```python
from build123d import *

# Parameters (mm, degrees)
F1_DEPTH = 25.4
F2_R     = 3.429
F3_DEPTH = 147.32
F4_W     = 22.8622798618
F4_H     = 12.7
F5_DEPTH = 25.4
F6_DEPTH = 76.2
F8_DEPTH = 25.4
F9_R     = 5.08


with BuildPart() as f1:
    # F0 (on Front) → F1 (new body)
    with BuildSketch(Plane.XZ):
        with BuildLine():
            Line((-25.4, 124.5236706513), (-25.4, 91.1413904513))
            Line((-25.4, 91.1413904513), (-25.4, -91.1413904513))
            Line((-25.4, -91.1413904513), (-25.4, -91.4211095487))
            Line((-25.4, -91.4211095487), (-25.4, -129.4763404513))
            Line((-25.4, -129.4763404513), (-2.5377201382, -129.4763404513))
            Line((-2.5377201382, -129.4763404513), (-2.5377201382, -103.8838730506))
            ThreePointArc((-2.5377201382, -103.8838730506), (-9.8366418496, -99.4730864008), (-12.7, -91.44))
            Line((-12.7, -91.44), (-12.7, 91.44))
            ThreePointArc((-12.7, 91.44), (-9.8366418496, 99.4730864008), (-2.5377201382, 103.8838730506))
            Line((-2.5377201382, 103.8838730506), (-2.5377201382, 124.5236706513))
            Line((-2.5377201382, 124.5236706513), (-25.4, 124.5236706513))
        make_face()
    extrude(amount=F1_DEPTH)

    # F2 (on face) → F3 (cut)
    with BuildSketch(Plane.YZ.offset(-2.5377201382)):
        with Locations((-12.7, -110.2338730506)):
            Circle(F2_R)
        with Locations((-12.7, 110.2338730506)):
            Circle(F2_R)
    extrude(amount=-F3_DEPTH, mode=Mode.SUBTRACT)

    # F4 (on face) → F5 (join)
    with BuildSketch(Plane.XZ.offset(25.4)):
        with Locations((-13.9688600691, -123.1263404513)):
            Rectangle(F4_W, F4_H)
    extrude(amount=F5_DEPTH)

    # F6 (add): a face of the model
    f6_faces = [f1.faces().sort_by_distance(p)[0] for p in [
        (-13.9688600691, -50.8, -123.1263404513),
    ]]
    extrude(f6_faces, amount=-F6_DEPTH)

    # F7 (on face) → F8 (cut)
    with BuildSketch(Plane.XY.offset(-116.7763404513)):
        with BuildLine():
            Line((-13.9688600691, 9.271), (-13.9688600691, 16.129))
            ThreePointArc((-13.9688600691, 16.129), (-17.3978600691, 12.7), (-13.9688600691, 9.271))
        make_face()
        with BuildLine():
            ThreePointArc((-10.5398600691, -38.1), (-11.5441909164, -35.6753308473), (-13.9688600691, -34.671))
            ThreePointArc((-13.9688600691, -34.671), (-16.3935292218, -40.5246691527), (-10.5398600691, -38.1))
        make_face()
        with BuildLine():
            ThreePointArc((-13.9688600691, 9.271), (-11.5441909164, 10.2753308473), (-10.5398600691, 12.7))
            ThreePointArc((-10.5398600691, 12.7), (-11.5441909164, 15.1246691527), (-13.9688600691, 16.129))
            Line((-13.9688600691, 16.129), (-13.9688600691, 9.271))
        make_face()
    extrude(amount=-F8_DEPTH, mode=Mode.SUBTRACT)

    # F9
    f9_edges = [f1.edges().sort_by_distance(p)[0] for p in [
        (-13.96886, -25.4, 124.523671),
        (-25.4, -12.7, 124.523671),
        (-13.96886, 0, 124.523671),
        (-25.4, -25.4, 3.873665),
        (-25.4, 0, 3.873665),
        (-13.96886, 0, -116.77634),
        (-13.96886, 25.4, -116.77634),
        (-25.4, -38.1, -116.77634),
        (-25.4, 12.7, -116.77634),
        (-25.4, 25.4, -123.12634),
        (-13.96886, -25.4, -116.77634),
        (-25.4, -50.8, -123.12634),
        (-13.96886, -50.8, -116.77634),
    ]]
    fillet(f9_edges, radius=F9_R)


solid = f1.part
```
Input: part model. Units: mm. Frame: model coordinates. A direction names the side the tool comes from. Coordinates: 2 decimals unless noted, no trailing zeros. Loops run counter-clockwise (first coordinate to the right, second up) from the corner with the lowest first, then second, coordinate; pieces in that order, holes last. Notation, with made-up numbers: M -13.75,-20.5 L 44.25,-20.5 A22 ccw 44.25,-7.5 Z; hole C -24.75,88.25 d9. An arc over 180 degrees is marked long. One line per item, written item: value.
(1) Reachability of faces 5 (the cylindrical face through (-23.951, -23.872, 2.256)), 6 (the flat face through (-16, -25.4, 5)), 7 (the cylindrical face through (-9.759, -12.522, -99.567)) from +Z, -Z, +X, -X, +Y, -Y: full face, straight path, thin tool, end or side. Return the list, or none.
Filled in:
face 5: +Z, -X, -Y
face 6: +Z, +X, -X, -Y
face 7: +X, +Y, -Y
(2) Section C-C (z = -74). Output: boundary loops of the cut face in (x, y), and give its area (3 significant figures).
Filled in:
outline: M -25.4,-20.32 A5.08 ccw -20.32,-25.4 L -12.7,-25.4 L -12.7,0 L -20.32,0 A5.08 ccw -25.4,-5.08 Z
area: 312 mm^2
(3) Section B-B (x = -8.25). Output: boundary loops of the cut face in (y, z), and give its area (3 significant figures).
Filled in:
outline: M -50.8,-129.48 L 25.4,-129.48 L 25.4,-121.86 A5.08 ccw 20.32,-116.78 L 5.08,-116.78 A5.08 cw 0,-111.7 L 0,-101.1 L -25.4,-101.1 L -25.4,-111.7 A5.08 cw -30.48,-116.78 L -45.72,-116.78 A5.08 ccw -50.8,-121.86 Z; M -25.4,101.1 L 0,101.1 L 0,119.44 A5.08 ccw -5.08,124.52 L -20.32,124.52 A5.08 ccw -25.4,119.44 Z; hole C -12.7,-110.23 d6.86; hole C -12.7,110.23 d6.86
area: 1,880 mm^2
(4) Pull-direction query (Z, two-part tool) for faces 1 (the flat face through (-25.4, -13, -15)), 2 (the flat face through (-14, -13, -129.476)), 3 (the flat face through (-12.7, -13, -1)), 4 (the cylindrical face through (-23.95, -12.81, 123)); classes: +Z half, -Z half, draft (parallel to the pull), parting line (faces both ways), or undercut.
Filled in:
face 1: draft
face 2: -Z half
face 3: undercut
face 4: +Z half
(5) Line query: line 1 along Z through (x, y) = (-16, -12.7); line 2 along X through (y, z) = (-38.1, -124.25); line 3 along Y through (x, z) = (-19.75, -36). Output: solid intervals per line, ascending. Write a range as from..to.
Filled in:
line 1: -129.48..-113.66, -106.8..106.8, 113.66..124.52
line 2: -25.4..-17.4, -10.54..-2.54
line 3: -25.4..0
(6) Section A-A (y = -12.7). Output: boundary loops of the cut face in (x, z).
Filled in:
outline: M -25.4,-129.48 L -2.54,-129.48 L -2.54,-113.66 L -25.4,-113.66 Z; M -25.4,-106.8 L -2.54,-106.8 L -2.54,-103.88 A12.7 cw -12.7,-91.44 L -12.7,91.44 A12.7 cw -2.54,103.88 L -2.54,106.8 L -25.4,106.8 Z; M -25.4,113.66 L -2.54,113.66 L -2.54,124.52 L -20.32,124.52 A5.08 ccw -25.4,119.44 Z
(7) Pin query (flat end, axial travel): pin 1 (4 mm diameter, centred on x = -17.5, y = -25.5, fed in from +Z); pin 2 (5.5 mm diameter, centred on x = -13, z = 26.5, fed in from -Y); pin 3 (2 mm diameter, centred on x = -9.5, y = -40.5, fed in from +Z); pin 4 (8 mm diameter, centred on y = -12.7, z = -110.23, fed in from +X). Return the tip coordinate at first contact, or that it passes through.
Filled in:
pin 1: z = 123.41
pin 2: y = -25.4
pin 3: z = -116.78
pin 4: x = -2.54
